```python
from build123d import *

# Parameters (mm, degrees)
F0_R     = 7.5
F1_DEPTH = 6
F2_R     = 2
F3_DEPTH = 12
F4_R     = 2.3
F5_DEPTH = 2
F7_DEPTH = 1


with BuildPart() as f1:
    # F0 (on Front) → F1 (new body)
    with BuildSketch(Plane.XZ):
        Circle(F0_R)
    extrude(amount=F1_DEPTH)

    # F2 (on face) → F3 (join)
    with BuildSketch(Plane.XZ.offset(6)):
        Circle(F2_R)
    extrude(amount=F3_DEPTH)

    # F4 (on face) → F5 (cut)
    with BuildSketch(Plane(origin=(0, 0, 0), x_dir=(-1, 0, 0), z_dir=(0, 1, 0))):
        with Locations((-4.5, 0)):
            Circle(F4_R)
        with Locations((4.5, 0)):
            Circle(F4_R)
    extrude(amount=-F5_DEPTH, mode=Mode.SUBTRACT)

    # F6 (on face) → F7 (cut)
    with BuildSketch(Plane.XZ.offset(6)):
        with BuildLine():
            Line((0.5, 3.5), (0.5, 7.4833147735))
            ThreePointArc((0.5, 7.4833147735), (0, 7.5), (-0.5, 7.4833147735))
            Line((-0.5, 7.4833147735), (-0.5, 3.5))
            ThreePointArc((-0.5, 3.5), (0, 3), (0.5, 3.5))
        make_face()
    extrude(amount=-F7_DEPTH, mode=Mode.SUBTRACT)


solid = f1.part
```
Source: CAD feature listing. Evaluate the final solid. Frame: model axes, mm. A direction names the side the tool comes from. Coordinates: 2 decimals unless noted, no trailing zeros. Write each loop counter-clockwise with the first axis right and the second up, starting at its lowest first coordinate (ties: lowest second). Pieces come first, ordered by that corner, then holes. Notation, with made-up numbers: M 67.25,8 L 88.25,8 A19 cw 88.25,35 Z; hole C 37.25,30 d5. An arc over 180 degrees is marked long. Answer as a JSON object with one key per item and string values.
1. Ray query, L1, parallel to Y at x = -3.5, z = -1; L2, parallel to Z at x = -4.5, y = -1.05; L3, parallel to Y at x = -0.25, z = 7.25. Return the intervals inside material, ascending.
Evaluation:
{"L1": "-6 to -2", "L2": "-6 to -2.3, 2.3 to 6", "L3": "-5 to 0"}
2. Cut plane C-C on x = 0. Output: boundary loops of the cut face in (y, z), plus the area to 4 significant figures.
Evaluation:
{"outline": "M -18,-2 L -6,-2 L -6,-7.5 L 0,-7.5 L 0,7.5 L -5,7.5 L -5,3 L -6,3 L -6,2 L -18,2 Z", "area": "133.5 mm^2"}
3. Cut plane D-D on y = -5.5. Output: boundary loops of the cut face in (x, z).
Evaluation:
{"outline": "M -0.5,3.5 L -0.5,7.48 A7.5 ccw long 0.5,7.48 L 0.5,3.5 A0.5 cw Z"}
4. Access query for faces 1 (the cylindrical face through (-7.493, -2.958, 0.33)), 2 (the flat face through (-0.5, -5.5, 5.5)), 3 (the flat face through (-4, -2, 0)). Directions: +Z, -Z, +X, -X, +Y, -Y. A direction counts if a zero-diameter tool reaches every point of the face in a straight line with its end or side. Return the directions, or none.
Evaluation:
{"face 1": "+Y, -Y", "face 2": "+Z, -Y", "face 3": "+Y"}
5. Draft query along X for faces 4 (the flat face through (0, -5, 5)), 5 (the flat face through (2, -6, -2)), 6 (the cylindrical face through (0, -12, -2)). Return one class per face: released by +X, released by -X, zero draft, split by the parting line, or undercut.
Evaluation:
{"face 4": "undercut", "face 5": "zero draft", "face 6": "split by the parting line"}
6. Cut plane A-A on x = 4.5. Output: boundary loops of the cut face in (y, z), plus the area to 3 significant figures.
Evaluation:
{"outline": "M -6,-6 L 0,-6 L 0,-2.3 L -2,-2.3 L -2,2.3 L 0,2.3 L 0,6 L -6,6 Z", "area": "62.8 mm^2"}
7. Cut plane B-B on z = 0. Output: boundary loops of the cut face in (x, y), plus the area to 3 significant figures.
Evaluation:
{"outline": "M -7.5,-6 L -2,-6 L -2,-18 L 2,-18 L 2,-6 L 7.5,-6 L 7.5,0 L 6.8,0 L 6.8,-2 L 2.2,-2 L 2.2,0 L -2.2,0 L -2.2,-2 L -6.8,-2 L -6.8,0 L -7.5,0 Z", "area": "120 mm^2"}
8. Contact query for flat-ended pins moving along their axis: P1, Ø8, axis at x = 1.5, y = -13.5, coming from the -Z side; P2, Ø1, axis at x = 5.5, z = 4, coming from the -Y side; P3, Ø3, axis at x = -4.5, z = 0, coming from the +Y side. Output: stop coordinate, or through.
Evaluation:
{"P1": "z = -2", "P2": "y = -6", "P3": "y = -2"}
